For this review, use the dimensioned drawing (mm, ordinates from the lowest corner) and the shaded views. A direction names the side the tool comes from. Give positions to 0.01 mm unless a question says otherwise; leave off trailing zeros. Order: outer loops, then holes, each group sorted by start corner. A loop starts at its lowest first (then second) coordinate and runs counter-clockwise, first axis right, second up. Notation, with made-up numbers: (-18, -7.5) - (36, -7.5) arc R27 ccw to (36, 18.5) - close; hole circle Ø1 at (72.25, -39.5). An arc over 180 degrees is marked (long way). Use a Markdown table: item, result. Add a question column.
1) We need section B-B on z = 15. Write out the cut boundary in (x, y).
2) Mouldability with a two-part tool opening along X and no side actions: class the marked faces 3, 4 and 5 as released by +X, released by -X, zero draft, split by the parting line, or undercut.
3) We need section A-A on x = 48.5. Write out the cut boundary in (y, z).
4) Machinability: for the marked faces 1 and 2, which of the approach directions +Z, -Z, +X, -X, +Y, -Y give a long, thin tool a straight path to every point of the face, cutting with its end or side? Answer none if there is none.
5) Wall thickness on L1, parallel to X at y = 6, z = 5.5; L2, parallel to X at y = 8, z = 15.75; L3, parallel to X at y = 4, z = 20: over which ranges is each line inside the solid? List them lowest first.
6) We need section D-D on z = 2. Write out the cut boundary in (x, y).
7) Clearance check with flat-ended pins moving along their axes: P1, Ø6.5, axis at x = 58.5, y = 6, coming from the +Z side; P2, Ø2.5, axis at x = 7, y = 6, coming from the +Z side. State where each tip first meets the part, or that it passes through.
8) We need section C-C on x = 6.5. Write out the cut boundary in (y, z), then the cut area to 3 significant figures.
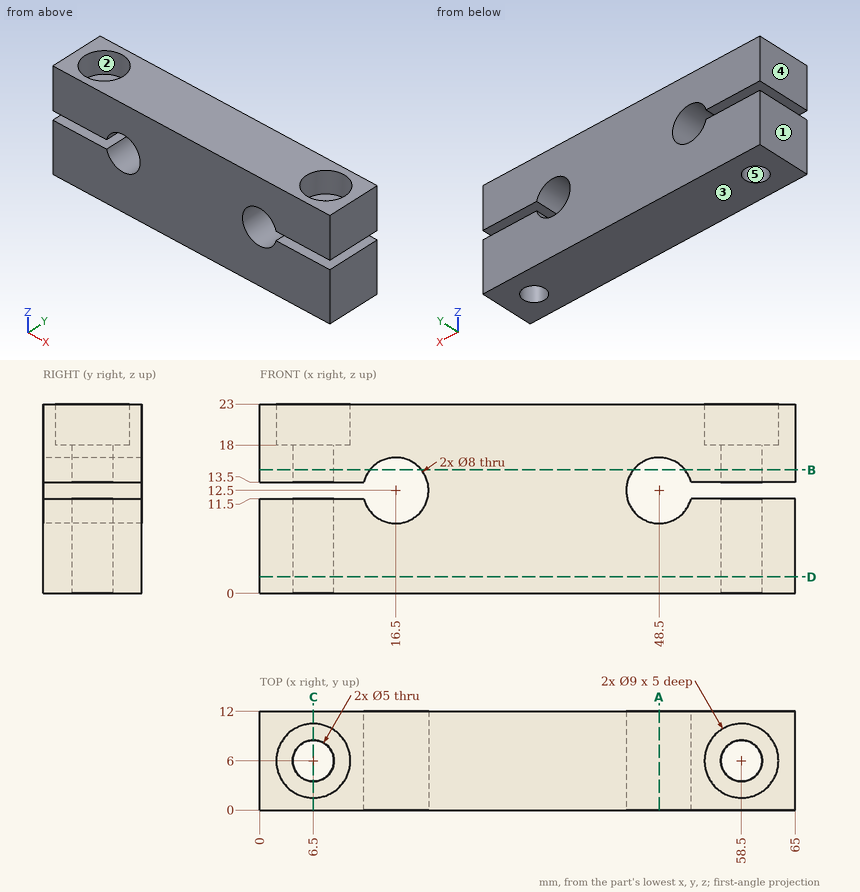
Checked values:
| question | item | result |
|---|---|---|
| 1 | outline | (0, 0) - (13.38, 0) - (13.38, 12) - (0, 12) - close; (19.62, 0) - (45.38, 0) - (45.38, 12) - (19.62, 12) - close; (51.62, 0) - (65, 0) - (65, 12) - (51.62, 12) - close; hole circle Ø5 at (6.5, 6); hole circle Ø5 at (58.5, 6) |
| 2 | face 3 | zero draft |
| 2 | face 4 | released by -X |
| 2 | face 5 | undercut |
| 3 | outline | (0, 0) - (12, 0) - (12, 8.5) - (0, 8.5) - close; (0, 16.5) - (12, 16.5) - (12, 23) - (0, 23) - close |
| 4 | face 1 | +Z, -Z, -X, +Y, -Y |
| 4 | face 2 | +Z |
| 5 | L1 | 0 to 4, 9 to 56, 61 to 65 |
| 5 | L2 | 0 to 5, 8 to 14.17, 18.83 to 46.17, 50.83 to 57, 60 to 65 |
| 5 | L3 | 0 to 2.47, 10.53 to 54.47, 62.53 to 65 |
| 6 | outline | (0, 0) - (65, 0) - (65, 12) - (0, 12) - close; hole circle Ø5 at (6.5, 6); hole circle Ø5 at (58.5, 6) |
| 7 | P1 | z = 18 |
| 7 | P2 | through |
| 8 | outline | (0, 0) - (3.5, 0) - (3.5, 11.5) - (0, 11.5) - close; (0, 13.5) - (3.5, 13.5) - (3.5, 18) - (1.5, 18) - (1.5, 23) - (0, 23) - close; (8.5, 0) - (12, 0) - (12, 11.5) - (8.5, 11.5) - close; (8.5, 13.5) - (12, 13.5) - (12, 23) - (10.5, 23) - (10.5, 18) - (8.5, 18) - close |
| 8 | area | 127 mm² |
